Check sheet for the modelled part. Datum: model origin and axes. Units: mm. Round coordinates to 2 decimals unless told otherwise and drop trailing zeros. Order: outer loops, then holes, each group sorted by start corner. A loop starts at its lowest first (then second) coordinate and runs counter-clockwise, first axis right, second up. Notation, with made-up numbers: (5, 32) -> (27, 32) arc R20 ccw to (27, 49) -> close; hole circle Ø4 at (-9.75, -37). An arc over 180 degrees is marked (long way). Answer in a Markdown table with one row per item.
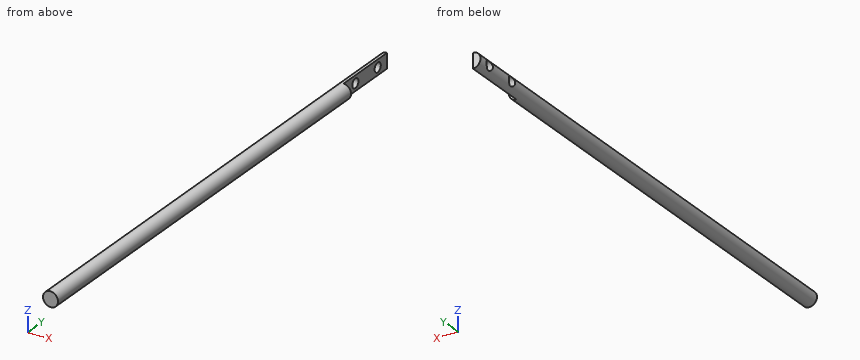
Autodesk Inventor part; units mm, degrees
ref_plane "YZ Plane" through (0, 0, 0) normal (1, 0, 0) x (0, 1, 0)
ref_plane "XZ Plane" through (0, 0, 0) normal (0, 1, 0) x (-1, 0, 0)
ref_plane "XY Plane" through (0, 0, 0) normal (0, 0, 1) x (1, 0, 0)
sketch "Sketch1" plane through (0, 0, 0) normal (0, 1, 0) x (-1, 0, 0)
  circle A0 centre (0, 0) radius 4
  dimension "d0" = 8
extrude "Extrusion1" add sketch "Sketch1" along normal blind 271.1467
sketch "Sketch2" plane through (0, 0, 0) normal (1, 0, 0) x (0, 1, 0)
  line L0 (-54.2293, 0) -> (325.3761, 0)
  line L1 (271.1467, -4) -> (271.1467, 4)
  line L2 (0, 4) -> (271.1467, 4)
  line L3 (271.1467, -4) -> (236.1467, -4)
  line L4 (236.1467, -4) -> (236.1467, 4)
  line L5 (236.1467, 4) -> (271.1467, 4)
  line L6 (271.1467, 4) -> (271.1467, -4)
  point P0 (0, 0)
  point P1 (263.6467, 0)
  point P2 (245.6467, 0)
  dimension "d4" = 7.5
  dimension "d5" = 18
  dimension "d6" = 35
extrude "Extrusion2" cut sketch "Sketch2" along normal blind 5
hole "Hole1" at (0, 263.6467, 0) at (0, 245.6467, 0) direction (-1, 0, 0) diameter 5 end through all
properties part number "bar" material "Stainless Steel"
(1) Section check A-A on z = 0. Record the boundary of the cut face in (x, y), plus the area to 3 significant figures.
Solutions:
| item | result |
|---|---|
| outline | (-4, 0) -> (4, 0) -> (4, 236.15) -> (0, 236.15) -> (0, 243.15) -> (-4, 243.15) -> close; (-4, 248.15) -> (0, 248.15) -> (0, 261.15) -> (-4, 261.15) -> close; (-4, 266.15) -> (0, 266.15) -> (0, 271.15) -> (-4, 271.15) -> close |
| area | 1,990 mm^2 |
(2) Scan lines: probe 1 along Y at (x, z) = (-2.3, 0); probe 2 along Y at (x, z) = (2.25, -1.25); probe 3 along X at (y, z) = (90, -0.25). Record each from-to range of solid material in increasing order. Write a range as from..to.
Solutions:
| item | result |
|---|---|
| probe 1 | 0..243.15, 248.15..261.15, 266.15..271.15 |
| probe 2 | 0..236.15 |
| probe 3 | -3.99..3.99 |
(3) Section check C-C on y = 206. Record the boundary of the cut face in (x, z), plus the area to 3 significant figures.
Solutions:
| item | result |
|---|---|
| outline | circle Ø8 at (0, 0) |
| area | 50.3 mm^2 |
(4) Section check B-B on x = -1.5. Record the boundary of the cut face in (y, z), plus the area to 3 significant figures.
Solutions:
| item | result |
|---|---|
| outline | (0, -3.71) -> (271.15, -3.71) -> (271.15, 3.71) -> (0, 3.71) -> close; hole circle Ø5 at (245.65, 0); hole circle Ø5 at (263.65, 0) |
| area | 1,970 mm^2 |
(5) Depth check by flat-ended pin: pin 1 Ø4 at (y, z) = (248.5, 0.5) entering from +X; pin 2 Ø1.2 at (x, z) = (1, -1) entering from +Y; pin 3 Ø1.5 at (x, y) = (-2.5, 93.5) entering from -Z. Enter the tip coordinate at first touch or a pass-through.
Solutions:
| item | result |
|---|---|
| pin 1 | x = 0 |
| pin 2 | y = 236.15 |
| pin 3 | z = -3.6 |
